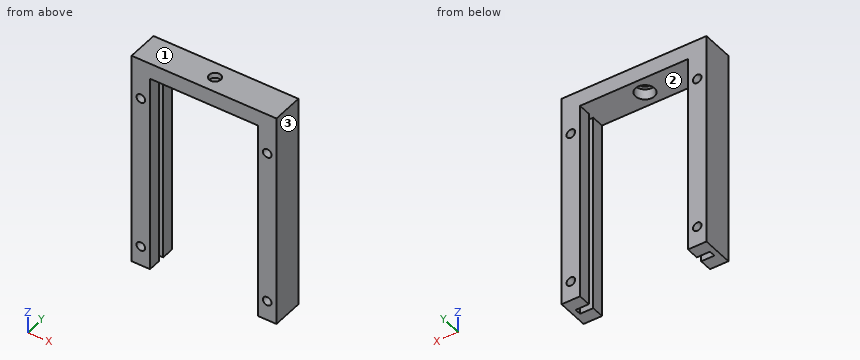
from build123d import *

# Parameters (mm, degrees)
F0_W      = 55
F0_H      = 12
F1_DEPTH  = 6
F2_D      = 4.4
F4_DEPTH  = 76
F6_D      = 3.3
F7_D      = 3.3
F8_D      = 3.3
F9_D      = 3.3
F10_R     = 3.6
F10_R_2   = 2.2
F11_DEPTH = 4


with BuildPart() as f1:
    # F0 (on Top) → F1 (new body)
    with BuildSketch(Plane.XY):
        Rectangle(F0_W, F0_H)
    extrude(amount=-F1_DEPTH)

    # F2 (through all)
    with Locations(Plane.XY):
        with Locations((0, 0)):
            Hole(F2_D / 2)

    # F3 (on face) → F4 (join)
    with BuildSketch(Plane(origin=(0, 0, -6), x_dir=(1, 0, 0), z_dir=(0, 0, -1))):
        Polygon((-20.5, 6), (-27.5, 6), (-27.5, -6), (-20.5, -6), (-20.5, -1.2), (-25.5, -1.2), (-25.5, 1.2), (-20.5, 1.2), align=None)
        Polygon((27.5, 6), (20.5, 6), (20.5, 1.2), (25.5, 1.2), (25.5, -1.2), (20.5, -1.2), (20.5, -6), (27.5, -6), align=None)
    extrude(amount=F4_DEPTH)

    # F6 (through all)
    with Locations(Plane(origin=(0, 6, 0), x_dir=(-1, 0, 0), z_dir=(0, 1, 0))):
        with Locations((24, -74.5)):
            Hole(F6_D / 2)

    # F7 (through all)
    with Locations(Plane(origin=(0, 6, 0), x_dir=(-1, 0, 0), z_dir=(0, 1, 0))):
        with Locations((-24, -74.5)):
            Hole(F7_D / 2)

    # F8 (through all)
    with Locations(Plane(origin=(0, 6, 0), x_dir=(-1, 0, 0), z_dir=(0, 1, 0))):
        with Locations((24, -15.5)):
            Hole(F8_D / 2)

    # F9 (through all)
    with Locations(Plane(origin=(0, 6, 0), x_dir=(-1, 0, 0), z_dir=(0, 1, 0))):
        with Locations((-24, -15.5)):
            Hole(F9_D / 2)

    # F10 (on face) → F11 (cut)
    with BuildSketch(Plane(origin=(0, 0, -6), x_dir=(1, 0, 0), z_dir=(0, 0, -1))):
        Circle(F10_R)
        Circle(F10_R_2, mode=Mode.SUBTRACT)
    extrude(amount=-F11_DEPTH, mode=Mode.SUBTRACT)


solid = f1.part
Can you work these out from the model? Positions are in its coordinate system, mm. Face numbers are marked on the shaded views. Coordinates: 2 decimals unless noted, no trailing zeros. Order: outer loops, then holes, each group sorted by start corner. A loop starts at its lowest first (then second) coordinate and runs counter-clockwise, first axis right, second up. Notation, with made-up numbers: (33.5, 53) - (79.5, 53) arc R30 ccw to (79.5, 77) - close; hole circle Ø4 at (-35.5, 48.5). An arc over 180 degrees is marked (long way). Answer as a JSON object with one key per item and string values. Group by question number.
Q1. We'd pull the mould along Z, two halves only. Please class the marked faces 1, 2 and 3: +Z half, -Z half, draft (parallel to the pull), parting line (faces both ways), or undercut.
Q2. Imagine slicing it at C-C (x = 24). Please give me the cut outline in (y, z).
Q3. I need wall thicknesses on line 1 (Z direction, x = -24, y = -3.25); line 2 (Z direction, x = 25.5, y = 2); line 3 (X direction, y = -4.75, z = -26). Which ranges of each line are inside material? Lowest first, please. Write a range as from..to.
Q4. Imagine slicing it at A-A (x = 0). Please give me the cut outline in (y, z), and give its area (3 significant figures).
Q5. Will this pin go through, and if not, where does the flat tip stop? P1, Ø4, axis at x = 0, y = 0, coming from the -Z side.
Q6. Imagine slicing it at B-B (z = -42.5). Please give me the cut outline in (x, y), and give its area (3 significant figures).
Q7. Imagine slicing it at D-D (z = -5). Please give me the cut outline in (x, y), and give its area (3 significant figures).
Determined:
{
 "1": {"face 1": "+Z half", "face 2": "-Z half", "face 3": "draft"},
 "2": {"outline": "(-6, -82) - (-1.2, -82) - (-1.2, -76.15) - (-6, -76.15) - close; (-6, -72.85) - (-1.2, -72.85) - (-1.2, -17.15) - (-6, -17.15) - close; (-6, -13.85) - (-1.2, -13.85) - (-1.2, -6) - (1.2, -6) - (1.2, -13.85) - (6, -13.85) - (6, 0) - (-6, 0) - close; (1.2, -82) - (6, -82) - (6, -76.15) - (1.2, -76.15) - close; (1.2, -72.85) - (6, -72.85) - (6, -17.15) - (1.2, -17.15) - close"},
 "3": {"line 1": "z = -82..-76.15, -72.85..-17.15, -13.85..0", "line 2": "z = -82..-75.19, -73.81..-16.19, -14.81..0", "line 3": "x = -27.5..-20.5, 20.5..27.5"},
 "4": {"outline": "(-6, -6) - (-3.6, -6) - (-3.6, -2) - (-2.2, -2) - (-2.2, 0) - (-6, 0) - close; (2.2, -2) - (3.6, -2) - (3.6, -6) - (6, -6) - (6, 0) - (2.2, 0) - close", "area": "34.4 mm2"},
 "5": {"P1": "passes through"},
 "6": {"outline": "(-27.5, -6) - (-20.5, -6) - (-20.5, -1.2) - (-25.5, -1.2) - (-25.5, 1.2) - (-20.5, 1.2) - (-20.5, 6) - (-27.5, 6) - close; (20.5, -6) - (27.5, -6) - (27.5, 6) - (20.5, 6) - (20.5, 1.2) - (25.5, 1.2) - (25.5, -1.2) - (20.5, -1.2) - close", "area": "144 mm2"},
 "7": {"outline": "(-27.5, -6) - (27.5, -6) - (27.5, 6) - (-27.5, 6) - close; hole circle Ø7.2 at (0, 0)", "area": "619 mm2"}
}
